Check sheet for the modelled part. Datum: model origin and axes. Units: mm. A direction names the side the tool comes from. Give positions to 0.01 mm unless a question says otherwise; leave off trailing zeros. Write each loop counter-clockwise with the first axis right and the second up, starting at its lowest first coordinate (ties: lowest second). Pieces come first, ordered by that corner, then holes. Notation, with made-up numbers: M 47,25 L 76,25 A16 cw 76,54 Z; hole C 27.25,87.5 d4. An arc over 180 degrees is marked long. Write item = value, one per line. Start each with the question number.
1) Gauge pin test, flat ends, axial feed: pin 1 (8 mm diameter, centred on x = 0, z = 0, fed in from -Y); pin 2 (3 mm diameter, centred on y = 9.5, z = 5.5, fed in from +X); pin 3 (3 mm diameter, centred on y = 7.5, z = -2.5, fed in from +X); pin 4 (10 mm diameter, centred on x = -8, z = -1.5, fed in from +Y). Record the tip position at first contact, or that the pin passes through.
2) Sectioned sample at A-A, the plane z = 0. Record the cut outline in (x, y).
3) Draft check along X on faces 3 (the face through (-15, 4, 10)), 4 (the face through (-1.08, 2.46, 4.88)), 5 (the face through (-10, 10, -7)), 6 (the face through (-25, 7, 0)). Enter one of: pulls with the +X half, pulls with the -X half, needs draft (parallel to the pull), parting line crosses it, or undercut.
4) Sectioned sample at B-B, the plane y = 11.5. Record the cut outline in (x, z).
5) Set-up check for faces 1 (the face through (-18, 15, -8)), 2 (the face through (-14.93, 8.959, 2.395)): record each of +Z, -Z, +X, -X, +Y, -Y from which the full face is reachable in a straight line by a thin tool's end or side.
6) Sectioned sample at C-C, the plane y = 2.5. Record the cut outline in (x, z).
7) Sectioned sample at D-D, the plane x = -22. Record the cut outline in (y, z).
8) Scan lines: L1, parallel to X at y = 3.9, z = 0; L2, parallel to Y at x = -18.5, z = 8.75; L3, parallel to X at y = 10.5, z = -7.75. Record each from-to range of solid material in increasing order.
from build123d import *

# Parameters (mm, degrees)
SKETCH_1_R          = 5
EXTRUDE_1_DEPTH     = 5
SKETCH_1_3_W        = 15
SKETCH_1_3_H        = 5
SKETCH_1_3_H_2      = 15
EXTRUDE_2_DEPTH     = 15
CUT_EXTRUDE_1_DEPTH = 15
CUT_EXTRUDE_2_DEPTH = 10


with BuildPart() as part:
    # Sketch 1 → Extrude 1 (new body)
    with BuildSketch(Plane(origin=(0, 0, 0), x_dir=(1, 0, 0), z_dir=(0, 1, 0))):
        with BuildLine():
            ThreePointArc((0, -10), (10, 0), (0, 10))
            Line((0, 10), (-10, 10))
            Line((-10, 10), (-10, 5))
            Line((-10, 5), (-10, -10))
            Line((-10, -10), (0, -10))
        make_face()
        Circle(SKETCH_1_R, mode=Mode.SUBTRACT)
    extrude(amount=EXTRUDE_1_DEPTH)

    # Sketch 1_3 → Extrude 2 (add)
    with BuildSketch(Plane(origin=(0, 0, 0), x_dir=(1, 0, 0), z_dir=(0, 1, 0))):
        with Locations((-17.5, 7.5)):
            Rectangle(SKETCH_1_3_W, SKETCH_1_3_H)
        with Locations((-17.5, -2.5)):
            Rectangle(SKETCH_1_3_W, SKETCH_1_3_H_2)
    extrude(amount=EXTRUDE_2_DEPTH)

    # Sketch 3 → Cut-Extrude 1 (cut)
    with BuildSketch(Plane(origin=(-10, 0, 0), x_dir=(0, 0, -1), z_dir=(1, 0, 0))):
        Polygon((5, 15), (-10, 10), (-10, 15), align=None)
    extrude(amount=-CUT_EXTRUDE_1_DEPTH, mode=Mode.SUBTRACT)

    # Sketch 2 → Cut-Extrude 2 (cut)
    with BuildSketch(Plane(origin=(0, 15, 0), x_dir=(1, 0, 0), z_dir=(0, 1, 0))):
        Polygon((-10, 5), (-20, -10), (-10, -10), align=None)
    extrude(amount=-CUT_EXTRUDE_2_DEPTH, mode=Mode.SUBTRACT)


solid = part.part
Data:
q1.pin_1 = through
q1.pin_2 = -16
q1.pin_3 = -10.67
q1.pin_4 = 15
q2.outline = M -25,0 L -5,0 L -5,5 L -13.33,5 L -13.33,13.33 L -25,13.33 Z; M 5,0 L 10,0 L 10,5 L 5,5 Z
q3.face_3 = needs draft
q3.face_4 = undercut
q3.face_5 = pulls with the +X half
q3.face_6 = pulls with the -X half
q4.outline = M -25,-10 L -10,-10 L -10,-5 L -17,5.5 L -25,5.5 Z
q5.face_1 = +Z, -Z, +X, -X, +Y
q5.face_2 = +Z, +X, +Y
q6.outline = M -25,-10 L 0,-10 A10 ccw 0,10 L -25,10 Z; hole C 0,0 d10
q7.outline = M 0,-10 L 15,-10 L 15,-5 L 10,10 L 0,10 Z
q8.L1 = -25 to -5, 5 to 10
q8.L2 = 0 to 5
q8.L3 = -25 to -10
